For this review, take the finished solid that the model builds, in its own axes (mm). Face numbers are marked on the shaded views. A direction names the side the tool comes from. Coordinates: 2 decimals unless noted, no trailing zeros. Write each loop counter-clockwise with the first axis right and the second up, starting at its lowest first coordinate (ties: lowest second). Pieces come first, ordered by that corner, then holes. Notation, with made-up numbers: (3.25, 63.5) - (22.25, 63.5) arc R24 ccw to (22.25, 87.5) - close; hole circle Ø1 at (-13.75, 11). An arc over 180 degrees is marked (long way). Use one line per item in the form item = value. Start each with the question number.
1) For L1, parallel to Z at x = -28.5, y = 22.5; L2, parallel to Z at x = -30, y = -9.5; L3, parallel to Y at x = -28, z = 15, list the stretches that pass through material, from the lowest coordinate up. Write a range as from..to.
2) We need section C-C (y = 52.5). Give the boundary of the cut face in (x, z).
3) We need section B-B (z = -11.5). Give the boundary of the cut face in (x, y).
4) We need section A-A (x = 9.5). Give the boundary of the cut face in (y, z).
5) Tool access review of the marked faces 4, 5, 6 and 7: name each direction out of +Z, -Z, +X, -X, +Y, -Y from which nothing blocks a thin tool from reaching the whole face with its end or side.
6) Insertion check: P1, Ø8, axis at x = -25, z = 9, coming from the +Y side; P2, Ø14, axis at x = 33.5, y = -8.5, coming from the +Z side; P3, Ø9, axis at y = -11.5, z = 14, coming from the +X side. Each pin has a flat end and moves straight along its axis. Give the tip position at first contact, or say it passes through.
7) We need section D-D (x = 26.5). Give the boundary of the cut face in (y, z), plus the area to 3 significant figures.
8) Mouldability with a two-part tool opening along Y and no side actions: class the marked faces 1, 2 and 3 as pulls with the +Y half, pulls with the -Y half, needs draft (parallel to the pull), parting line crosses it, or undercut.
```python
from build123d import *

# Parameters (mm, degrees)
F1_DEPTH = 17.78
F2_W     = 101.6
F2_H     = 17.78
F3_DEPTH = 38.1
F4_DEPTH = 38.1
F6_R     = 22.4750173509
F7_DEPTH = 50.8
F8_DEPTH = 50.8
F9_DEPTH = 50.8


with BuildPart() as f1:
    # F0 (on Front) → F1 (new body)
    with BuildSketch(Plane.XZ):
        Polygon((-38.1, -25.4), (38.1, -25.4), (38.1, 7.62), (20.32, 7.62), (20.32, 25.4), (-38.1, 25.4), align=None)
    extrude(amount=F1_DEPTH)

    # F2 (on Right) → F3 (join)
    with BuildSketch(Plane.YZ):
        with Locations((50.8, -16.759835723)):
            Rectangle(F2_W, F2_H)
    extrude(amount=F3_DEPTH)

    # F4 (add): a face of the model
    f4_faces = [f1.faces().sort_by_distance(p)[0] for p in [
        (0, 50.8, -16.759835723),
    ]]
    extrude(f4_faces, amount=F4_DEPTH)

    # F6 (on Top) → F7 (cut)
    with BuildSketch(Plane.XY):
        with Locations((0, 63.0396232009)):
            Circle(F6_R)
    extrude(amount=-F7_DEPTH, mode=Mode.SUBTRACT)

    # F5 (on face) → F8 (cut)
    with BuildSketch(Plane.XY.offset(-7.869835723)):
        with BuildLine():
            ThreePointArc((1.241e-07, 101.6), (26.9407684071, 90.4407683193), (38.1, 63.5))
            Line((38.1, 63.5), (38.1, 101.6))
            Line((38.1, 101.6), (1.241e-07, 101.6))
        make_face()
    extrude(amount=-F8_DEPTH, mode=Mode.SUBTRACT)

    # F5 (on face) → F9 (cut)
    with BuildSketch(Plane.XY.offset(-7.869835723)):
        with BuildLine():
            ThreePointArc((-38.1, 63.5), (-26.9407683193, 90.4407684071), (1.241e-07, 101.6))
            Line((1.241e-07, 101.6), (-38.1, 101.6))
            Line((-38.1, 101.6), (-38.1, 63.5))
        make_face()
    extrude(amount=-F9_DEPTH, mode=Mode.SUBTRACT)


solid = f1.part
```
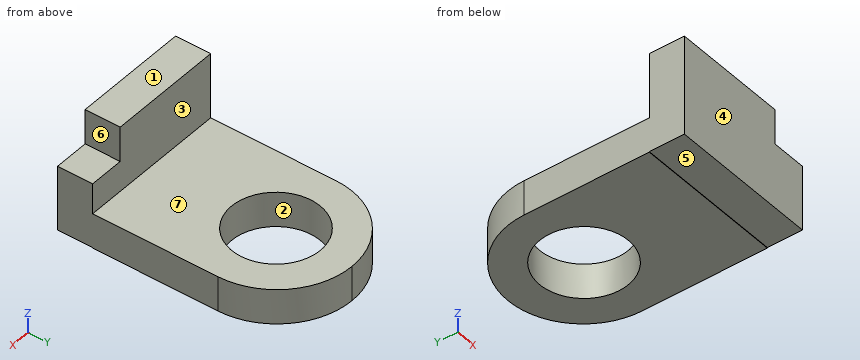
Determined:
q1.L1 = -25.65..-7.87
q1.L2 = -25.4..25.4
q1.L3 = -17.78..0
q2.outline = (-38.1, -25.65) - (-19.85, -25.65) - (-19.85, -7.87) - (-38.1, -7.87) - close; (19.85, -25.65) - (38.1, -25.65) - (38.1, -7.87) - (19.85, -7.87) - close
q3.outline = (-38.1, -17.78) - (38.1, -17.78) - (38.1, 63.5) arc R38.1 ccw to (-38.1, 63.5) - close; hole circle Ø44.95 at (0, 63.04)
q4.outline = (-17.78, -25.4) - (0, -25.4) - (0, -25.65) - (42.67, -25.65) - (42.67, -7.87) - (0, -7.87) - (0, 25.4) - (-17.78, 25.4) - close; (83.41, -25.65) - (100.4, -25.65) - (100.4, -7.87) - (83.41, -7.87) - close
q5.face_4 = +Z, -Z, +X, -X, -Y
q5.face_5 = -Z, +X, -X, -Y
q5.face_6 = +Z, +X, +Y, -Y
q5.face_7 = +Z, +X, -X, +Y
q6.P1 = 0
q6.P2 = 7.62
q6.P3 = 20.32
q7.outline = (-17.78, -25.4) - (0, -25.4) - (0, -25.65) - (90.87, -25.65) - (90.87, -7.87) - (0, -7.87) - (0, 7.62) - (-17.78, 7.62) - close
q7.area = 2,200 mm²
q8.face_1 = needs draft
q8.face_2 = undercut
q8.face_3 = pulls with the +Y half
